Input: dimensioned drawing with shaded views. Units: mm. Origin: part minimum x, y, z. Coordinates: 2 decimals unless noted, no trailing zeros. Loops run counter-clockwise (first coordinate to the right, second up) from the corner with the lowest first, then second, coordinate; pieces in that order, holes last.
Item 1: Ray query, line 1 along Y through (x, z) = (10, 3.55); line 2 along Y through (x, z) = (10, 0.5); line 3 along X through (y, z) = (11.5, 3.35). Return the intervals inside material, ascending.
Item 2: Pull-direction query (X, two-part tool) for the marked faces 1, 2 and 3; classes: released by +X, released by -X, zero draft, split by the parting line, or undercut.
Item 3: Contact query for flat-ended pins moving along their axis: P1, Ø1, axis at y = 16, z = 4, coming from the -X side; P2, Ø5.5, axis at x = 10, y = 10, coming from the +Z side; P3, Ø2, axis at y = 8.5, z = 4, coming from the +X side. Output: stop coordinate, or through.
Item 4: Section A-A on x = 10. Return loops of the section in (y, z), and give its area (3 significant figures).
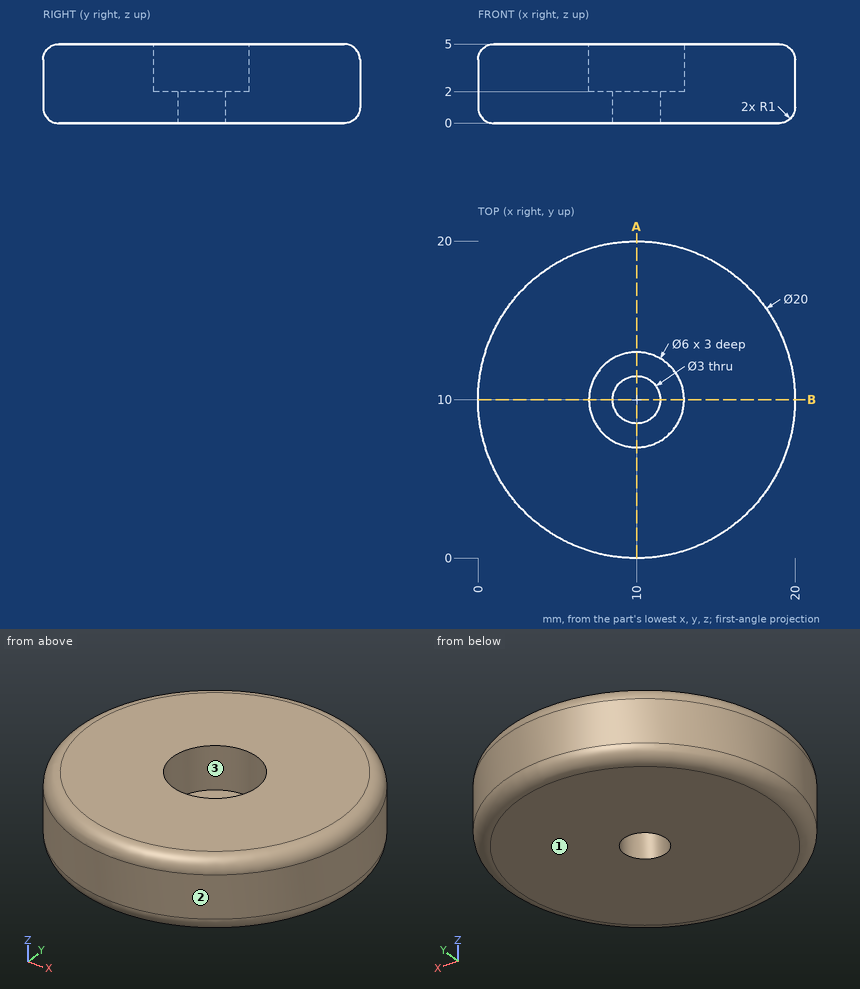
Results found:
1. line 1: y = 0 to 7, 13 to 20
1. line 2: y = 0.13 to 8.5, 11.5 to 19.87
1. line 3: x = 0.11 to 7.4, 12.6 to 19.89
2. face 1: zero draft
2. face 2: split by the parting line
2. face 3: undercut
3. P1: stops at x = 1.65
3. P2: stops at z = 2
3. P3: stops at x = 19.99
4. outline: (0, 1) arc R1 ccw to (1, 0) - (8.5, 0) - (8.5, 2) - (7, 2) - (7, 5) - (1, 5) arc R1 ccw to (0, 4) - close; (11.5, 0) - (19, 0) arc R1 ccw to (20, 1) - (20, 4) arc R1 ccw to (19, 5) - (13, 5) - (13, 2) - (11.5, 2) - close
4. area: 75.1 mm2
